Check sheet for the modelled part. Datum: model origin and axes. Units: mm. Face numbers are marked on the shaded views. A direction names the side the tool comes from. Round coordinates to 2 decimals unless told otherwise and drop trailing zeros. Order: outer loops, then holes, each group sorted by start corner. A loop starts at its lowest first (then second) coordinate and runs counter-clockwise, first axis right, second up.
(1) Depth check by flat-ended pin: pin 1 (0.9 mm diameter, centred on x = 64.5, y = 2, fed in from +Z); pin 2 (3.5 mm diameter, centred on x = -64.5, y = 1, fed in from +Z); pin 3 (3 mm diameter, centred on y = 0, z = 17.5, fed in from +X). Enter the tip coordinate at first touch or a pass-through.
(2) Mould release check, pull along Z, two halves, no side actions. Record for the marked faces 1 and 2: released by +Z, released by -Z, zero draft, split by the parting line, or undercut.
(3) Sectioned sample at D-D, the plane z = -35. Enter the section's corners in (x, y), and give its area (3 significant figures).
(4) Tool access check on the marked faces 3, 4 and 5. Record the directions out of +Z, -Z, +X, -X, +Y, -Y that give a thin tool (end or side, any length) a straight path to the whole face; none if there is none.
(5) Sectioned sample at A-A, the plane y = -14. Enter the section's corners in (x, z).
(6) Sectioned sample at B-B, the plane x = -28. Enter the section's corners in (y, z).
(7) Thickness scan on probe 1 along Z at (x, y) = (60.25, -4.4); probe 2 along X at (y, z) = (-7, 5); probe 3 along Y at (x, z) = (-60.2, 0). Record the ranges inside material, lowest first.
(8) Sectioned sample at C-C, the plane z = 8.5. Enter the section's corners in (x, y), and give its area (3 significant figures).
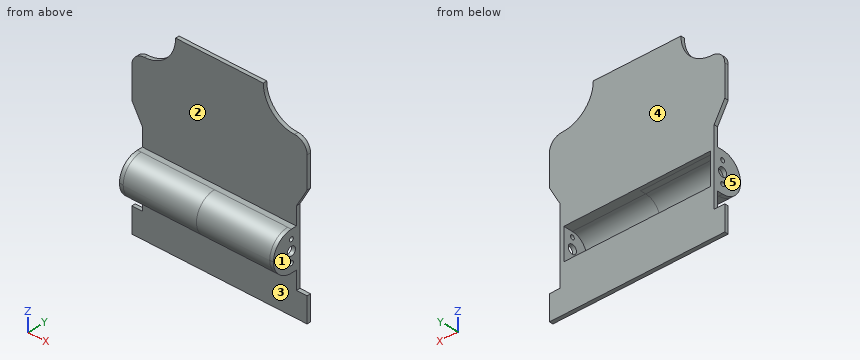
Autodesk Inventor part; units mm, degrees
ref_plane "YZ Plane" through (0, 0, 0) normal (1, 0, 0) x (0, 1, 0)
ref_plane "XZ Plane" through (0, 0, 0) normal (0, 1, 0) x (-1, 0, 0)
ref_plane "XY Plane" through (0, 0, 0) normal (0, 0, 1) x (1, 0, 0)
sketch "Sketch1" plane through (0, 0, 0) normal (0, 1, 0) x (-1, 0, 0)
  line L0 (70, 45) -> (61.5, 30)
  line L1 (61.5, 30) -> (61.5, -30)
  line L2 (61.5, -30) -> (70, -30)
  line L3 (70, -30) -> (70, -50)
  line L4 (70, -50) -> (-70, -50)
  line L5 (-70, -50) -> (-70, -30)
  line L6 (-70, -30) -> (-61.5, -30)
  line L7 (-61.5, -30) -> (-61.5, 30)
  line L8 (-61.5, 30) -> (-70, 45)
  line L9 (70, 45) -> (70, 80)
  line L10 (-70, 45) -> (-70, 80)
  line L11 (35, 105) -> (-35, 105)
  line L12 (-98, 0) -> (98, 0)
  line L13 (0, -81) -> (0, 136)
  line L14 (70, 80) -> (35, 80)
  line L15 (35, 80) -> (35, 105)
  line L16 (-35, 105) -> (-35, 80)
  line L17 (-35, 80) -> (-70, 80)
  point P0 (0, 0)
  dimension "d0" = 60
  dimension "d1" = 60
  dimension "d2" = 123
  dimension "d3" = 140
  dimension "d4" = 20
  dimension "d5" = 140
  dimension "d8" = 35
  dimension "d15" = 30
  dimension "d45" = 15
  dimension "d46" = 15
  dimension "d47" = 35
  dimension "d48" = 70
  dimension "d49" = 155
extrude "Extrusion1" add sketch "Sketch1" along normal blind 3
sketch "Sketch2" plane through (0, 0, 0) normal (0, -1, 0) x (1, 0, 0)
  line L0 (-98, 0) -> (98, 0)
  line L1 (0, 136) -> (0, -81)
  line L2 (61.5, 15.6) -> (58.5, 15.6)
  line L3 (58.5, 15.6) -> (58.5, -15.6)
  line L4 (58.5, -15.6) -> (61.5, -15.6)
  line L5 (61.5, -15.6) -> (61.5, 15.6)
  line L6 (61.5, 30) -> (61.5, -30)
  point P0 (0, 0)
  dimension "d18" = 3
  dimension "d19" = 31.2
extrude "Extrusion2" add sketch "Sketch2" along normal blind 20
sketch "Sketch3" plane through (61.5, 0, -30) normal (1, 0, 0) x (0, 0, -1)
  line L0 (-45.6, 0) -> (-45.6, -20)
  line L1 (-14.4, -20) -> (-45.6, -20)
  line L2 (-30, -24.6) -> (-30, 7.6)
  point P0 (-30, 0)
  point P1 (-38.5, -4.4)
  point P2 (-21.5, -4.4)
  dimension "d22" = 17
  dimension "d23" = 15.6
hole "Hole1" at (61.5, -4.4, 8.5) at (61.5, -4.4, -8.5) direction (-1, 0, 0) diameter 3.4 end through all
sketch "Sketch4" plane through (61.5, 0, -30) normal (1, 0, 0) x (0, 0, -1)
  line L0 (-30, -24.6) -> (-30, 7.6)
  circle A0 centre (-38.5, -4.4) radius 1.7
  circle A1 centre (-21.5, -4.4) radius 1.7
  line L1 (-38.5, -4.4) -> (-21.5, -4.4) construction
  point P0 (-30, 0)
  point P1 (-30, -4.4)
hole "Hole2" at (61.5, -4.4, 0) direction (-1, 0, 0) diameter 7.1 end through all
fillet "Fillet1" radius 15.6 2 edges at (60, -20, -15.6) (60, -20, 15.6)
sketch "Sketch5" plane through (0, 0, 0) normal (1, 0, 0) x (0, 1, 0)
  line L0 (-24, 0) -> (4, 0)
  circle A0 centre (-4.4, 0) radius 3.55
  arc A1 (-4.4, 12.6) -> (-4.4, -12.6) centre (-4.4, 0) ccw
  arc A2 (-4.4, 15.6) -> (-4.4, -15.6) centre (-4.4, 0) ccw
  line L1 (0, -15.6) -> (-4.4, -15.6)
  line L2 (-4.4, -15.6) -> (0, -15.6)
  line L3 (0, 30) -> (0, 15.6)
  line L4 (0, 15.6) -> (-4.4, 15.6)
  line L5 (-4.4, 15.6) -> (0, 15.6)
  line L6 (0, -15.6) -> (0, 15.6)
  line L7 (0, 15.6) -> (0, -15.6)
  line L8 (-4.4, 12.6) -> (0, 12.6)
  line L9 (-4.4, -12.6) -> (0, -12.6)
  point P0 (0, 0)
  point P1 (0, -12.6)
  point P2 (0, 12.6)
  dimension "d39" = 25.2
  dimension "d40" = 3
extrude "Extrusion3" add sketch "Sketch5" along normal up to surface (58.5 mm away) contours A2 L4 L6 L8 A1 L0 | L0 A1 L9 L6 L1 A2
sketch "Sketch6" plane through (0, 0, 0) normal (1, 0, 0) x (0, 1, 0)
  line L0 (0, 42) -> (0, -42)
  line L1 (-5.88, 0) -> (4.48, 0)
  line L2 (3, 12.6) -> (0, 12.6)
  line L3 (0, 12.6) -> (0, -12.6)
  line L4 (0, -12.6) -> (3, -12.6)
  line L5 (3, -12.6) -> (3, 12.6)
  line L6 (0, -12.6) -> (-4.4, -12.6)
  line L7 (-4.4, 12.6) -> (0, 12.6)
  line L8 (3, -30) -> (3, 30)
  line L9 (0, -30) -> (0, 30)
  point P0 (0, 0)
  point P1 (0, 12.6)
  point P2 (0, -12.6)
extrude "Extrusion4" cut sketch "Sketch6" along normal mid plane 117
mirror "Mirror1" about plane through (0, 0, 0) normal (1, 0, 0) of "Hole1", "Hole2", "Extrusion2", "Fillet1", "Extrusion3"
fillet "Fillet2" radius 25 2 edges at (35, 1.5, 80) (-35, 1.5, 80)
fillet "Fillet3" radius 10 2 edges at (70, 1.5, 80) (-70, 1.5, 80)
properties part number "karoserie1"
Derived:
1. pin 1: stops at z = 79.14
1. pin 2: stops at z = 79.61
1. pin 3: stops at x = 61.5
2. face 1: undercut
2. face 2: zero draft
3. outline: (-70, 0) - (70, 0) - (70, 3) - (-70, 3) - close
3. area: 420 mm2
4. face 3: -Z, +X, -X, -Y
4. face 4: +Z, -Z, +X, -X, +Y
4. face 5: -X, +Y, -Y
5. outline: (-61.5, -12.3) - (61.5, -12.3) - (61.5, 12.3) - (-61.5, 12.3) - close; hole (-58.5, -8.16) - (58.5, -8.16) - (58.5, 8.16) - (-58.5, 8.16) - close
6. outline: (-4.4, -15.6) - (0, -15.6) - (0, -50) - (3, -50) - (3, -12.6) - (-4.4, -12.6) arc R12.6 cw to (-4.4, 12.6) - (3, 12.6) - (3, 105) - (0, 105) - (0, 15.6) - (-4.4, 15.6) arc R15.6 ccw to start
7. probe 1: z = -15.6 to -10.2, -6.8 to -3.55, 3.55 to 6.8, 10.2 to 15.6
7. probe 2: x = -61.5 to -58.5, 58.5 to 61.5
7. probe 3: y = -20 to -7.95, -0.85 to 3
8. outline: (-61.5, -17.48) - (61.5, -17.48) - (61.5, -6.1) - (58.5, -6.1) - (58.5, -13.7) - (-58.5, -13.7) - (-58.5, -6.1) - (-61.5, -6.1) - close; (-61.5, -2.7) - (-58.5, -2.7) - (-58.5, 3) - (-61.5, 3) - close; (58.5, -2.7) - (61.5, -2.7) - (61.5, 3) - (58.5, 3) - close
8. area: 545 mm2
